```python
from build123d import *

# Parameters (mm, degrees)
F0_R     = 20.6945995874
F1_DEPTH = 25.4
F2_T     = -2.54


# Not quite as in the source:
# - a fillet or chamfer that OpenCascade refuses, or shapes differently, is made with other operations: its cross-section is extruded or revolved along the edge and cut away or added


with BuildPart() as f1:
    # F0 (on Top) → F1 (new body)
    with BuildSketch(Plane.XY):
        Circle(F0_R)
    extrude(amount=F1_DEPTH)

    # F2
    f2_openings = [f1.faces().sort_by_distance(p)[0] for p in [
        (0, 0, 25.4),
    ]]
    offset(amount=F2_T, openings=f2_openings)

    # F3: fillet of radius 5.08 on 1 edges, made by hand

    # F3_s1 → F3_t2 (revolve, cut)
    with BuildSketch(Plane.XZ):
        with BuildLine():
            ThreePointArc((20.6945995874, 21.0005909488), (20.0140086386, 23.5405909488), (18.1545995874, 25.4))
            Line((18.1545995874, 25.4), (20.6945995874, 25.4))
            Line((20.6945995874, 25.4), (20.6945995874, 21.0005909488))
        make_face()
    revolve(axis=Axis((0, 0, 25.4), (0, 0, 1)), mode=Mode.SUBTRACT)


solid = f1.part
```
Work out the finished part from the listing and answer in its coordinate system (mm). Round coordinates to 2 decimals unless told otherwise and drop trailing zeros. Order: outer loops, then holes, each group sorted by start corner. A loop starts at its lowest first (then second) coordinate and runs counter-clockwise, first axis right, second up.
Q1. The mould has two halves that part along Y. Classify faces 1 (the flat face through (0, 0, 2.54)), 2 (the flat face through (0, 0, 0)), 3 (the cylindrical face through (-16.423, -12.592, 10.353)): pulls with the +Y half, pulls with the -Y half, needs draft (parallel to the pull), parting line crosses it, or undercut.
Solution:
face 1: undercut
face 2: needs draft
face 3: parting line crosses it
Q2. Find the intervals of material crossed by line 1 along Y through (x, z) = (0, 18); line 2 along Z through (x, y) = (-5.5, -5.5); line 3 along X through (y, z) = (-5.5, 7.5), in increasing order.
Solution:
line 1: y = -20.69 to -18.15, 18.15 to 20.69
line 2: z = 0 to 2.54
line 3: x = -19.95 to -17.3, 17.3 to 19.95
Q3. A cutting plane is placed at D-D, the plane z = 2. Determine the outline of the cut face in (x, y), then the cut area to 3 significant figures.
Solution:
outline: circle Ø41.39 at (0, 0)
area: 1,350 mm2
Q4. A cutting plane is placed at B-B, the plane y = 0. Determine the outline of the cut face in (x, z).
Solution:
outline: (-20.69, 0) - (20.69, 0) - (20.69, 21) arc R5.08 ccw to (18.15, 25.4) - (18.15, 2.54) - (-18.15, 2.54) - (-18.15, 25.4) arc R5.08 ccw to (-20.69, 21) - close
Q5. Given pin 1 Ø2 at (y, z) = (-3.5, 20) entering from -X; pin 2 Ø22 at (x, y) = (0, 0) entering from +Z; pin 3 Ø4 at (x, z) = (-14, 7.5) entering from -Y, each flat-ended and moving along its own axis, determine where each tip first touches the part or whether it passes through.
Solution:
pin 1: stops at x = -20.54
pin 2: stops at z = 2.54
pin 3: stops at y = -16.86
Q6. A cutting plane is placed at A-A, the plane z = 20. Determine the outline of the cut face in (x, y), then the cut area to 3 significant figures.
Solution:
outline: circle Ø41.39 at (0, 0); hole circle Ø36.31 at (0, 0)
area: 310 mm2
